```python
from build123d import *

# Parameters (mm, degrees)
F0_R           = 12.5
F1_DEPTH       = 1
F2_R           = 6.2
F3_DEPTH       = 10
F4_R           = 12.7
F5_DEPTH       = 25
F5_DEPTH_BACK  = 25
F7_R           = 2
F8_DEPTH       = 10
F9_W           = 9.563760832
F9_H           = 3.8901750788
F10_DEPTH      = 12.501
F10_DEPTH_BACK = 12.501


with BuildPart() as f1:
    # F0 (on Top) → F1 (new body)
    with BuildSketch(Plane.XY):
        Circle(F0_R)
    extrude(amount=F1_DEPTH)

    # F2 (on face) → F3 (join)
    with BuildSketch(Plane(origin=(0, 0, 0), x_dir=(1, 0, 0), z_dir=(0, 0, -1))):
        Circle(F2_R)
    extrude(amount=F3_DEPTH)

    # F4 (on Front) → F5 (cut, two sides)
    with BuildSketch(Plane.XZ) as f5_sk:
        with Locations((0, -20)):
            Circle(F4_R)
    extrude(amount=-F5_DEPTH, mode=Mode.SUBTRACT)
    extrude(f5_sk.sketch, amount=F5_DEPTH_BACK, mode=Mode.SUBTRACT)

    # F7 (on offset) → F8 (cut, through all)
    with BuildSketch(Plane.XY.offset(-10)):
        Circle(F7_R)
    extrude(amount=F8_DEPTH, mode=Mode.SUBTRACT)

    # F9 (on Front) → F10 (cut, two sides)
    with BuildSketch(Plane.XZ) as f10_sk:
        with Locations((-4.781880416, -9.2450875394)):
            Rectangle(F9_W, F9_H)
    extrude(amount=-F10_DEPTH, mode=Mode.SUBTRACT)
    extrude(f10_sk.sketch, amount=F10_DEPTH_BACK, mode=Mode.SUBTRACT)


solid = f1.part
```
Geometry check sheet. Reference: the model listing, model coordinates, mm. A direction names the side the tool comes from. Coordinates: 2 decimals unless noted, no trailing zeros. Order: outer loops, then holes, each group sorted by start corner. A loop starts at its lowest first (then second) coordinate and runs counter-clockwise, first axis right, second up.
Q1. Sectioned sample at B-B on x = 5.25. Record the cut outline in (y, z), and give its area (3 significant figures).
Reply:
outline: (-11.34, 0) - (-3.3, 0) - (-3.3, -8.44) - (3.3, -8.44) - (3.3, 0) - (11.34, 0) - (11.34, 1) - (-11.34, 1) - close
area: 78.3 mm2
Q2. Sectioned sample at D-D on x = 1.25. Record the cut outline in (y, z), and give its area (3 significant figures).
Reply:
outline: (-12.44, 0) - (-6.07, 0) - (-6.07, -7.36) - (-1.56, -7.36) - (-1.56, 0) - (1.56, 0) - (1.56, -7.36) - (6.07, -7.36) - (6.07, 0) - (12.44, 0) - (12.44, 1) - (-12.44, 1) - close
area: 91.3 mm2
Q3. Thickness scan on probe 1 along X at (y, z) = (0, -2); probe 2 along Z at (x, y) = (-4, -11.5). Record the ranges inside material, lowest first.
Reply:
probe 1: x = -6.2 to -2, 2 to 6.2
probe 2: z = 0 to 1
Q4. Sectioned sample at A-A on y = 0. Record the cut outline in (x, z).
Reply:
outline: (-12.5, 0) - (-6.2, 0) - (-6.2, -7.3) - (-2, -7.3) - (-2, 0) - (2, 0) - (2, -7.46) arc R12.7 cw to (6.2, -8.92) - (6.2, 0) - (12.5, 0) - (12.5, 1) - (-12.5, 1) - close
Q5. Tool access check on faces 1 (the face through (5.9, -1.9, -3.4)), 2 (the face through (-3, 0, -7.3)), 3 (the face through (0, 0, 1)). Record the directions out of +Z, -Z, +X, -X, +Y, -Y that give a thin tool (end or side, any length) a straight path to the whole face; none if there is none.
Reply:
face 1: -Z
face 2: -Z, -X, +Y, -Y
face 3: +Z, +X, -X, +Y, -Y
Q6. Draft check along X on faces 4 (the face through (0, 0, 0)), 5 (the face through (3.247, -0.087, -7.722)), 6 (the face through (-6, -3, 0)), 7 (the face through (0, -2, -4)). Enter one of: released by +X, released by -X, zero draft, split by the parting line, or undercut.
Reply:
face 4: undercut
face 5: released by -X
face 6: zero draft
face 7: undercut
Q7. Depth check by flat-ended pin: pin 1 Ø1.5 at (x, z) = (4.5, -1.5) entering from +Y; pin 2 Ø4 at (x, y) = (3, 3.5) entering from -Z; pin 3 Ø1 at (y, z) = (2, -4.5) entering from -X. Enter the tip coordinate at first touch or a pass-through.
Reply:
pin 1: stops at y = 4.94
pin 2: stops at z = -8.33
pin 3: stops at x = -6.02
Q8. Sectioned sample at C-C on z = -5.25. Record the cut outline in (x, y), and give its area (3 significant figures).
Reply:
outline: circle Ø12.4 at (0, 0); hole circle Ø4 at (0, 0)
area: 108 mm2
